Here's how the part is built. I have some questions about the finished solid (model axes, mm). A direction names the side the tool comes from. Coordinates: 2 decimals unless noted, no trailing zeros. Order: outer loops, then holes, each group sorted by start corner. A loop starts at its lowest first (then second) coordinate and runs counter-clockwise, first axis right, second up. Notation, with made-up numbers: (77.5, 73.5) - (124.5, 73.5) arc R30 ccw to (124.5, 104.5) - close; hole circle Ø1 at (-34, 79.25). An arc over 180 degrees is marked (long way). Answer in a Markdown table with one row per item. Add a question column.
Item 1: I want a section at C-C (z = 0.8). Count the separate pieces of the cut face and the enclosed holes in it, plus the area to 3 significant figures.
Item 2: If I drill on line 1 along Y through (x, z) = (19.05, 0.8); line 2 along X through (y, z) = (-6.5, 3.2) (1 decimal); line 3 along X through (y, z) = (-6.5, 3.6) (1 decimal), over which ranges is the centre line in solid material (lowest first)? Write a range as from..to.
Item 3: Will these pins go through, and if not, where does the flat tip stop? pin 1 Ø1 at (x, y) = (-1, -4.5) entering from +Z; pin 2 Ø1.3 at (x, y) = (-35, -26) entering from +Z (3 decimals); pin 3 Ø0.5 at (x, z) = (-34, 2.5) entering from +Y; pin 4 Ø15.5 at (x, y) = (19.05, 0) entering from -Z.
Item 4: On a 3-axis mill with a long thin cutter (end or side, diameter ignored), from which of +Z, -Z, +X, -X, +Y, -Y can I reach the whole of each face in a straight line? I mean faces 1 (the flat face through (1, 0, 0)), 2 (the flat face through (-49.212, -9, 3)), 3 (the flat face through (-52, -6.35, 3)). Say none if no direction works.
Item 5: Thinking about a two-plate mould opening in X: for faces 4 (the flat face through (-35, -27, 2)), 5 (the cylindrical face through (-51.75, -5.44, 0.78)), 6 (the cylindrical face through (46.923, -21.835, 0.805)), 7 (the flat face through (49.212, -9, 3)), which applies, +X half, -X half, draft (parallel to the pull), parting line (faces both ways), or undercut?
Item 6: I want a section at A-A (y = 0). Please give me the cut outline in (x, z), plus the area to 3 significant figures.
Item 7: I want a section at D-D (y = 17.5). Please give me the cut outline in (x, z), plus the area to 3 significant figures.
Item 8: I want a section at B-B (x = -12.7). Please give me the cut outline in (y, z).
```python
from build123d import *

# Parameters (mm, degrees)
F0_W         = 101.6
F0_H         = 50.8
F0_R         = 1.905
F1_DEPTH     = 1.5875
F3_R         = 12.7
F4_R         = 2.54
F2_R         = 4.826
F2_R_2       = 1.905
F5_DEPTH     = 3.175
F6_W         = 6.35
F6_H         = 1.5875
F7_DEPTH     = 1.6002
F8_W         = 6.35
F8_H         = 1.5875
F9_DEPTH     = 1.6002
F10_W        = 6.35
F10_H        = 1.5875
F11_DEPTH    = 3.175
F12_W        = 6.35
F12_H        = 1.5875
F13_DEPTH    = 3.175
F14_W        = 6.35
F14_H        = 1.6002
F15_DEPTH    = 1.5875
F14_W_2      = 3.175
F14_H_2      = 6.35
F16_DEPTH    = 3.302
F17_W        = 6.35
F17_H        = 1.524
F18_DEPTH    = 1.5875
F19_W        = 6.35
F19_H        = 1.524
F20_DEPTH    = 1.5875
F21_T1_DEPTH = 1.5875
F22_W        = 0.254
F22_H        = 6.35
F23_DEPTH    = 2.032
F24_W        = 0.254
F24_H        = 6.35
F25_DEPTH    = 2.032


# Not quite as in the source:
# - a fillet or chamfer that OpenCascade refuses, or shapes differently, is made with other operations: its cross-section is extruded or revolved along the edge and cut away or added


with BuildPart() as f1:
    # F0 (on Top) → F1 (new body)
    with BuildSketch(Plane.XY):
        Rectangle(F0_W, F0_H)
        with Locations((-12.7, 0)):
            Circle(F0_R, mode=Mode.SUBTRACT)
        with Locations((19.05, 0)):
            Circle(F0_R, mode=Mode.SUBTRACT)
    extrude(amount=F1_DEPTH)

    # F3
    f3_edges = [f1.edges().sort_by_distance(p)[0] for p in [
        (-50.8, -25.4, 0.79375),
        (50.8, -25.4, 0.79375),
    ]]
    fillet(f3_edges, radius=F3_R)

    # F4
    f4_edges = [f1.edges().sort_by_distance(p)[0] for p in [
        (-50.8, 25.4, 0.79375),
        (50.8, 25.4, 0.79375),
    ]]
    fillet(f4_edges, radius=F4_R)

    # F2 (on face) → F5 (cut)
    with BuildSketch(Plane.XY.offset(1.5875)):
        with Locations((-12.7, 0)):
            Circle(F2_R)
        with Locations((-12.7, 0)):
            Circle(F2_R_2, mode=Mode.SUBTRACT)
        with Locations((19.05, 0)):
            Circle(F2_R)
        with Locations((19.05, 0)):
            Circle(F2_R_2, mode=Mode.SUBTRACT)
    extrude(amount=-F5_DEPTH, mode=Mode.SUBTRACT)

    # F6 (on face) → F7 (join)
    with BuildSketch(Plane(origin=(0, 25.4, 0), x_dir=(-1, 0, 0), z_dir=(0, 1, 0))):
        with Locations((-45.085, 0.79375)):
            Rectangle(F6_W, F6_H)
        with Locations((45.085, 0.79375)):
            Rectangle(F6_W, F6_H)
    extrude(amount=F7_DEPTH)

    # F8 (on face) → F9 (join)
    with BuildSketch(Plane.XZ.offset(25.4)):
        with Locations((34.925, 0.79375)):
            Rectangle(F8_W, F8_H)
        with Locations((-34.925, 0.79375)):
            Rectangle(F8_W, F8_H)
    extrude(amount=F9_DEPTH)

    # F10 (on face) → F11 (join)
    with BuildSketch(Plane(origin=(-50.8, 0, 0), x_dir=(0, -1, 0), z_dir=(-1, 0, 0))):
        with Locations((9.525, 0.79375)):
            Rectangle(F10_W, F10_H)
    extrude(amount=F11_DEPTH)

    # F12 (on face) → F13 (join)
    with BuildSketch(Plane.YZ.offset(50.8)):
        with Locations((-9.525, 0.79375)):
            Rectangle(F12_W, F12_H)
    extrude(amount=F13_DEPTH)

    # F14 (on face) → F15 (join)
    with BuildSketch(Plane.XY.offset(1.5875)):
        with Locations((45.085, 26.2001)):
            Rectangle(F14_W, F14_H)
        with Locations((34.925, -26.2001)):
            Rectangle(F14_W, F14_H)
        with Locations((-34.925, -26.2001)):
            Rectangle(F14_W, F14_H)
        with Locations((-45.085, 26.2001)):
            Rectangle(F14_W, F14_H)
    extrude(amount=F15_DEPTH)

    # F14 (on face) → F16 (join)
    with BuildSketch(Plane.XY.offset(1.5875)):
        with Locations((52.3875, -9.525)):
            Rectangle(F14_W_2, F14_H_2)
        with Locations((-52.3875, -9.525)):
            Rectangle(F14_W_2, F14_H_2)
    extrude(amount=F16_DEPTH)

    # F17 (on face) → F18 (join)
    with BuildSketch(Plane.YZ.offset(-50.8)):
        with Locations((-9.525, 4.1275)):
            Rectangle(F17_W, F17_H)
    extrude(amount=F18_DEPTH)

    # F19 (on face) → F20 (join)
    with BuildSketch(Plane(origin=(50.8, 0, 0), x_dir=(0, -1, 0), z_dir=(-1, 0, 0))):
        with Locations((9.525, 4.1275)):
            Rectangle(F19_W, F19_H)
    extrude(amount=F20_DEPTH)

    # F21: fillet of radius 3.175 on 12 edges, made by hand

    # F21_s2 → F21_t1 (join)
    with BuildSketch(Plane.XY):
        with BuildLine():
            ThreePointArc((-28.9930759967, -25.4), (-30.5869133472, -25.8290379646), (-31.75, -27.0002))
            Line((-31.75, -27.0002), (-31.75, -25.4))
            Line((-31.75, -25.4), (-28.9930759967, -25.4))
        make_face()
        with BuildLine():
            ThreePointArc((-38.1, -27.0002), (-39.0345990401, -25.8098604937), (-40.4140641084, -25.1873979396))
            ThreePointArc((-40.4140641084, -25.1873979396), (-39.2619049374, -25.3467377974), (-38.1, -25.4))
            Line((-38.1, -25.4), (-38.1, -27.0002))
        make_face()
        with BuildLine():
            ThreePointArc((-50.5434078933, -15.24), (-51.6462135525, -13.4156555752), (-53.6542598667, -12.7))
            Line((-53.6542598667, -12.7), (-50.8, -12.7))
            ThreePointArc((-50.8, -12.7), (-50.7356891432, -13.9764638175), (-50.5434078933, -15.24))
        make_face()
        with BuildLine():
            ThreePointArc((-53.975, -6.35), (-51.7299359697, -5.4200640303), (-50.8, -3.175))
            Line((-50.8, -3.175), (-50.8, -6.35))
            Line((-50.8, -6.35), (-53.975, -6.35))
        make_face()
        with BuildLine():
            ThreePointArc((-49.6405789052, 24.9920417178), (-48.7499512331, 25.8583913172), (-48.26, 27.0002))
            Line((-48.26, 27.0002), (-48.26, 25.4))
            ThreePointArc((-48.26, 25.4), (-48.9797965118, 25.2958762246), (-49.6405789052, 24.9920417178))
        make_face()
        with BuildLine():
            ThreePointArc((-41.91, 27.0002), (-40.7469133472, 25.8290379646), (-39.1530759967, 25.4))
            Line((-39.1530759967, 25.4), (-41.91, 25.4))
            Line((-41.91, 25.4), (-41.91, 27.0002))
        make_face()
        with BuildLine():
            ThreePointArc((48.26, 27.0002), (48.7499512331, 25.8583913172), (49.6405789052, 24.9920417178))
            ThreePointArc((49.6405789052, 24.9920417178), (48.9797965118, 25.2958762246), (48.26, 25.4))
            Line((48.26, 25.4), (48.26, 27.0002))
        make_face()
        with BuildLine():
            ThreePointArc((39.1530759967, 25.4), (40.7469133472, 25.8290379646), (41.91, 27.0002))
            Line((41.91, 27.0002), (41.91, 25.4))
            Line((41.91, 25.4), (39.1530759967, 25.4))
        make_face()
        with BuildLine():
            ThreePointArc((50.8, -3.175), (51.7299359697, -5.4200640303), (53.975, -6.35))
            Line((53.975, -6.35), (50.8, -6.35))
            Line((50.8, -6.35), (50.8, -3.175))
        make_face()
        with BuildLine():
            ThreePointArc((53.6542598667, -12.7), (51.6462135525, -13.4156555752), (50.5434078933, -15.24))
            ThreePointArc((50.5434078933, -15.24), (50.7356891432, -13.9764638175), (50.8, -12.7))
            Line((50.8, -12.7), (53.6542598667, -12.7))
        make_face()
        with BuildLine():
            ThreePointArc((40.4140641084, -25.1873979396), (39.0345990401, -25.8098604937), (38.1, -27.0002))
            Line((38.1, -27.0002), (38.1, -25.4))
            ThreePointArc((38.1, -25.4), (39.2619049374, -25.3467377974), (40.4140641084, -25.1873979396))
        make_face()
        with BuildLine():
            ThreePointArc((31.75, -27.0002), (30.5869133472, -25.8290379646), (28.9930759967, -25.4))
            Line((28.9930759967, -25.4), (31.75, -25.4))
            Line((31.75, -25.4), (31.75, -27.0002))
        make_face()
    extrude(amount=F21_T1_DEPTH)

    # F22 (on face) → F23 (join)
    with BuildSketch(Plane(origin=(0, 0, 3.3655), x_dir=(1, 0, 0), z_dir=(0, 0, -1))):
        with Locations((49.3395, 9.525)):
            Rectangle(F22_W, F22_H)
    extrude(amount=F23_DEPTH)

    # F24 (on face) → F25 (join)
    with BuildSketch(Plane(origin=(0, 0, 3.3655), x_dir=(1, 0, 0), z_dir=(0, 0, -1))):
        with Locations((-49.3395, 9.525)):
            Rectangle(F24_W, F24_H)
    extrude(amount=F25_DEPTH)


solid = f1.part
```
Values follow:
| question | item | result |
|---|---|---|
| 1 | separate pieces | 1 |
| 1 | enclosed holes | 2 |
| 1 | area | 5,040 mm^2 |
| 2 | line 1 | y = -25.4..-4.83, 4.83..25.4 |
| 2 | line 2 | x = -54..-50.8, -49.5..-49.2, 49.2..49.5, 50.8..54 |
| 2 | line 3 | x = -54..-49.2, 49.2..54 |
| 3 | pin 1 | stops at z = 1.59 |
| 3 | pin 2 | stops at z = 3.175 |
| 3 | pin 3 | stops at y = -25.4 |
| 3 | pin 4 | stops at z = 0 |
| 4 | face 1 | -Z, +X, -X, +Y, -Y |
| 4 | face 2 | +Z, +Y, -Y |
| 4 | face 3 | +Z, +X, -X, +Y |
| 5 | face 4 | draft |
| 5 | face 5 | -X half |
| 5 | face 6 | +X half |
| 5 | face 7 | undercut |
| 6 | outline | (-50.8, 0) - (-17.53, 0) - (-17.53, 1.59) - (-50.8, 1.59) - close; (-7.87, 0) - (14.22, 0) - (14.22, 1.59) - (-7.87, 1.59) - close; (23.88, 0) - (50.8, 0) - (50.8, 1.59) - (23.88, 1.59) - close |
| 6 | area | 131 mm^2 |
| 7 | outline | (-50.8, 0) - (50.8, 0) - (50.8, 1.59) - (-50.8, 1.59) - close |
| 7 | area | 161 mm^2 |
| 8 | outline | (-25.4, 0) - (-4.83, 0) - (-4.83, 1.59) - (-25.4, 1.59) - close; (4.83, 0) - (25.4, 0) - (25.4, 1.59) - (4.83, 1.59) - close |
